from build123d import *

# Parameters (mm, degrees)
SKETCH_W         = 25.5
SKETCH_H         = 62.15
PAD_DEPTH        = 4.6
THICKNESS_T      = 1.6
SKETCH001_R      = 2.5
PAD001_DEPTH     = 3.09
SKETCH002_R      = 1.6
POCKET_DEPTH     = 3
FILLET_R         = 0.8
SKETCH003_W      = 27.1
SKETCH003_H      = 63.75
SKETCH003_W_2    = 25.5
SKETCH003_H_2    = 62.15
PAD002_DEPTH     = 0.8
SKETCH004_W      = 9.39
SKETCH004_H      = 0.965
POCKET001_DEPTH  = 5
SKETCH005_R      = 2.5
PAD003_DEPTH     = 3.09
HOLE_D           = 2.4
HOLE_DEPTH       = 25
HOLE_CSINK_D     = 4
HOLE_CSINK_ANGLE = 90


with BuildPart() as part:
    # Sketch (on Face4132 of Binder) → Pad (new body)
    with BuildSketch(Plane.XY.offset(1.51)):
        with Locations((12.5, 27.925)):
            Rectangle(SKETCH_W, SKETCH_H)
    extrude(amount=-PAD_DEPTH)

    # Thickness
    thickness_openings = [part.faces().sort_by_distance(p)[0] for p in [
        (12.5, 27.925, 1.51),
    ]]
    offset(amount=THICKNESS_T, openings=thickness_openings, kind=Kind.INTERSECTION)

    # Sketch001 (on Face5 of Thickness) → Pad001 (join)
    with BuildSketch(Plane.XY.offset(-3.09)):
        with Locations((2.5, 0.5)):
            Circle(SKETCH001_R)
        with Locations((22.5, 0.5)):
            Circle(SKETCH001_R)
        with Locations((2.5, 50)):
            Circle(SKETCH001_R)
        with Locations((22.5, 50)):
            Circle(SKETCH001_R)
    extrude(amount=PAD001_DEPTH)

    # Sketch002 (on Face18 of Pad001) → Pocket (cut)
    with BuildSketch(Plane.XY):
        with Locations((2.5, 50)):
            Circle(SKETCH002_R)
        with Locations((22.5, 50)):
            Circle(SKETCH002_R)
        with Locations((2.5, 0.5)):
            Circle(SKETCH002_R)
        with Locations((22.5, 0.5)):
            Circle(SKETCH002_R)
    extrude(amount=-POCKET_DEPTH, mode=Mode.SUBTRACT)

    # Fillet
    fillet_edges = [part.edges().sort_by_distance(p)[0] for p in [
        (-1.85, -4.75, -1.59),
        (26.85, -4.75, -1.59),
        (-1.85, 60.6, -1.59),
        (26.85, 60.6, -1.59),
    ]]
    fillet(fillet_edges, radius=FILLET_R)

    # Sketch003 (on Face1 of Fillet) → Pad002 (join)
    with BuildSketch(Plane.XY.offset(1.51)):
        with Locations((12.5, 27.925)):
            Rectangle(SKETCH003_W, SKETCH003_H)
        with Locations((12.5, 27.925)):
            Rectangle(SKETCH003_W_2, SKETCH003_H_2, mode=Mode.SUBTRACT)
    extrude(amount=PAD002_DEPTH)

    # Sketch004 (on Face17 of Pad002) → Pocket001 (cut)
    with BuildSketch(Plane(origin=(0, -3.15, 0), x_dir=(-1, 0, 0), z_dir=(0, 1, 0))):
        with Locations((-12.525, 1.8275)):
            Rectangle(SKETCH004_W, SKETCH004_H)
    extrude(amount=-POCKET001_DEPTH, mode=Mode.SUBTRACT)

    # Sketch005 (on Face25 of Pocket001) → Pad003 (join)
    with BuildSketch(Plane.XY.offset(-3.09)):
        with Locations((2.5, 50)):
            Circle(SKETCH005_R)
        with Locations((22.5, 50)):
            Circle(SKETCH005_R)
        with Locations((2.5, 0.5)):
            Circle(SKETCH005_R)
        with Locations((22.5, 0.5)):
            Circle(SKETCH005_R)
    extrude(amount=PAD003_DEPTH)

    # Hole
    with Locations(Plane(origin=(0, 0, -4.69), x_dir=(1, 0, 0), z_dir=(0, 0, -1))):
        with Locations((2.5, -0.5), (22.5, -0.5), (2.5, -50), (22.5, -50)):
            CounterSinkHole(HOLE_D / 2, HOLE_CSINK_D / 2, depth=HOLE_DEPTH, counter_sink_angle=HOLE_CSINK_ANGLE)


solid = part.part
The model under review builds one solid part; all positions refer to its coordinate system, in mm. A direction names the side the tool comes from. Coordinates: 2 decimals unless noted, no trailing zeros. Write each loop counter-clockwise with the first axis right and the second up, starting at its lowest first coordinate (ties: lowest second). Pieces come first, ordered by that corner, then holes. Notation, with made-up numbers: (29.5, -7.75) - (37.5, -7.75) arc R27 ccw to (37.5, 25.25) - close; hole circle Ø10 at (21.5, 0.25). An arc over 180 degrees is marked (long way). Answer as a JSON object with one key per item and string values. Group by question number.
1. To check wall thickness, follow probe 1 along Y at (x, z) = (22.5, -2.15); probe 2 along X at (y, z) = (7.5, -2.5); probe 3 along Y at (x, z) = (24, -3). State the ranges of each line that lie inside material, in increasing order.
2. Add section D-D (x = 13.5). Give the boundary of the cut face in (y, z) (3 decimals).
3. Add section A-A (z = -2). Give the number of separate pieces and of enclosed holes in the cut face, plus the area to 3 significant figures.
4. Machinability: for faces 1 (the face through (20, 50, -2)), 2 (the face through (13, -4, 1.345)), 3 (the face through (12, -4.75, -2)), which of the approach directions +Z, -Z, +X, -X, +Y, -Y give a long, thin tool a straight path to every point of the face, cutting with its end or side? Answer none if there is none.
5. Mouldability with a two-part tool opening along X and no side actions: class faces 4 (the face through (24, 51, 0)), 5 (the face through (20, 0.6, -1.6)), 6 (the face through (25.5, 28.1, 2.31)) as pulls with the +X half, pulls with the -X half, needs draft (parallel to the pull), parting line crosses it, or undercut.
6. Clearance check with flat-ended pins moving along their axes: pin 1 Ø3 at (x, y) = (23, 31.5) entering from +Z; pin 2 Ø1.8 at (x, y) = (13.5, -4) entering from +Z (3 decimals); pin 3 Ø4 at (x, y) = (22, 51) entering from +Z. State where each tip first meets the part, or that it passes through.
Findings:
{
 "1": {"probe 1": "-4.75 to -3.15, -2 to -0.7, 1.7 to 3, 47.5 to 48.8, 51.2 to 52.5, 59 to 60.6", "probe 2": "-1.85 to -0.25, 25.25 to 26.85", "probe 3": "-4.75 to -3.15, -1.5 to 2.5, 48 to 52, 59 to 60.6"},
 "2": {"outline": "(-4.75, -4.69) - (60.6, -4.69) - (60.6, 1.51) - (59.8, 1.51) - (59.8, 2.31) - (59, 2.31) - (59, -3.09) - (-3.15, -3.09) - (-3.15, 1.345) - (-4.75, 1.345) - close"},
 "3": {"separate pieces": "5", "enclosed holes": "5", "area": "351 mm²"},
 "4": {"face 1": "+Z", "face 2": "+Z, -Y", "face 3": "+Z, -Z, +X, -X, -Y"},
 "5": {"face 4": "undercut", "face 5": "undercut", "face 6": "needs draft"},
 "6": {"pin 1": "z = -3.09", "pin 2": "z = 1.345", "pin 3": "z = 0"}
}
